```python
from build123d import *

# Parameters (mm, degrees)
SKETCH_R         = 33
PAD_DEPTH        = 37
SKETCH001_R      = 40.2
PAD001_DEPTH     = 5
SKETCH002_R      = 30
POCKET_DEPTH     = 37
HOLE_D           = 3.6
HOLE_DEPTH       = 5
HOLE_CBORE_D     = 6.2
HOLE_CBORE_DEPTH = 3
FILLET001_R      = 1.25
CHAMFER_SIZE     = 0.4


with BuildPart() as part:
    # Sketch → Pad (new body)
    with BuildSketch(Plane.XY):
        Circle(SKETCH_R)
    extrude(amount=PAD_DEPTH)

    # Sketch001 → Pad001 (join)
    with BuildSketch(Plane.XY):
        Circle(SKETCH001_R)
    extrude(amount=PAD001_DEPTH)

    # Sketch002 → Pocket (cut)
    with BuildSketch(Plane.XY):
        Circle(SKETCH002_R)
    extrude(amount=POCKET_DEPTH, mode=Mode.SUBTRACT)

    # Hole
    with Locations(Plane.XY.offset(5)):
        with Locations((-36.6, 0), (18.3, 31.69653), (18.3, -31.69653)):
            CounterBoreHole(HOLE_D / 2, HOLE_CBORE_D / 2, HOLE_CBORE_DEPTH, depth=HOLE_DEPTH)

    # Fillet001
    fillet001_edges = [part.edges().sort_by_distance(p)[0] for p in [
        (-33, 0, 37),
        (-30, 0, 37),
    ]]
    fillet(fillet001_edges, radius=FILLET001_R)

    # Chamfer
    chamfer_edges = [part.edges().sort_by_distance(p)[0] for p in [
        (-40.2, 0, 5),
        (-40.2, 0, 0),
    ]]
    chamfer(chamfer_edges, length=CHAMFER_SIZE)


solid = part.part
```
Model file for the job. Use its own axes, mm. A direction names the side the tool comes from. Coordinates: 2 decimals unless noted, no trailing zeros. Loops run counter-clockwise (first coordinate to the right, second up) from the corner with the lowest first, then second, coordinate; pieces in that order, holes last. Notation, with made-up numbers: (-24, 83.5) - (-2, 83.5) arc R24 ccw to (-2, 114.5) - close; hole circle Ø2 at (78.25, -35). An arc over 180 degrees is marked (long way). Write item = value, one per line. Start each with the question number.
Item 1: Drop flat-ended pins along their axis: pin 1 Ø7 at (x, y) = (-37.5, 1.5) entering from +Z; pin 2 Ø4 at (x, y) = (18.3, -31.7) entering from -Z; pin 3 Ø1.5 at (y, z) = (26.5, 16.5) entering from +X; pin 4 Ø1 at (x, z) = (1, 10) entering from -Y. Give the stop position or say it passes through.
Item 2: Saw through at B-B, the plane y = 0. List the corners of the cut face in (x, z).
Item 3: 3-axis set-ups, long thin cutter, end or side, ignore diameter. For faces 4 (the face through (-39.7, 0.1, 3.5)), 5 (the face through (18.69, 29.94, 0.99)): which of +Z, -Z, +X, -X, +Y, -Y reach the whole face in a straight line?
Item 4: Saw through at A-A, the plane x = 0. List the corners of the cut face in (y, z).
Item 5: Wall check: probe 1 along X at (y, z) = (-9, 17); probe 2 along X at (y, z) = (-0.5, 1); probe 3 along Y at (x, z) = (-26, 9). Give the ranges that are in metal, low to high. Write a range as [from, to].
Item 6: Pull direction X, two halves, no side cores. Call faces 1 (the face through (38.344, 12.075, 2.471)), 2 (the face through (18.53, -29.91, 0.99)), 3 (the face through (-9, -29, 0)): +X half, -X half, draft (parallel to the pull), parting line (faces both ways), or undercut.
Item 7: Saw through at C-C, the plane z = 32. List the corners of the cut face in (x, y), then the cut area to 3 significant figures.
Item 8: Saw through at D-D, the plane x = 18.3. State how many separate pieces and enclosed holes the cut face has, then the cut area to 3 significant figures.
Answers:
q1.pin_1 = 5
q1.pin_2 = 0
q1.pin_3 = 20.64
q1.pin_4 = -33
q2.outline = (-40.2, 0.4) - (-39.8, 0) - (-38.4, 0) - (-38.4, 2) - (-39.7, 2) - (-39.7, 5) - (-39.8, 5) - (-40.2, 4.6) - close; (-34.8, 0) - (-30, 0) - (-30, 35.75) arc R1.25 ccw to (-31.25, 37) - (-31.75, 37) arc R1.25 ccw to (-33, 35.75) - (-33, 5) - (-33.5, 5) - (-33.5, 2) - (-34.8, 2) - close; (30, 0) - (39.8, 0) - (40.2, 0.4) - (40.2, 4.6) - (39.8, 5) - (33, 5) - (33, 35.75) arc R1.25 ccw to (31.75, 37) - (31.25, 37) arc R1.25 ccw to (30, 35.75) - close
q3.face_4 = +Z
q3.face_5 = +Z, -Z
q4.outline = (-40.2, 0.4) - (-39.8, 0) - (-30, 0) - (-30, 35.75) arc R1.25 ccw to (-31.25, 37) - (-31.75, 37) arc R1.25 ccw to (-33, 35.75) - (-33, 5) - (-39.8, 5) - (-40.2, 4.6) - close; (30, 0) - (39.8, 0) - (40.2, 0.4) - (40.2, 4.6) - (39.8, 5) - (33, 5) - (33, 35.75) arc R1.25 ccw to (31.75, 37) - (31.25, 37) arc R1.25 ccw to (30, 35.75) - close
q5.probe_1 = [-31.75, -28.62], [28.62, 31.75]
q5.probe_2 = [-40.2, -38.33], [-34.87, -30], [30, 40.2]
q5.probe_3 = [-20.32, -14.97], [14.97, 20.32]
q6.face_1 = parting line
q6.face_2 = undercut
q6.face_3 = draft
q7.outline = circle Ø66 at (0, 0); hole circle Ø60 at (0, 0)
q7.area = 594 mm2
q8.separate_pieces = 4
q8.enclosed_holes = 0
q8.area = 303 mm2
